Autodesk Inventor part; units mm, degrees
ref_plane "YZ Plane" through (0, 0, 0) normal (1, 0, 0) x (0, 1, 0)
ref_plane "XZ Plane" through (0, 0, 0) normal (0, 1, 0) x (-1, 0, 0)
ref_plane "XY Plane" through (0, 0, 0) normal (0, 0, 1) x (1, 0, 0)
sketch "スケッチ1" plane through (0, 0, 0) normal (0, 0, 1) x (1, 0, 0)
  line L0 (14, 16) -> (-14, 16)
  line L1 (-16, 14) -> (-16, -14)
  line L2 (-14, -16) -> (14, -16)
  line L3 (16, -14) -> (16, 14)
  line L4 (16, 16) -> (-16, -16) construction
  line L5 (-16, 16) -> (16, -16) construction
  line L6 (-13, 13) -> (13, 13) construction
  line L7 (13, 13) -> (13, -13) construction
  line L8 (13, -13) -> (-13, -13) construction
  line L9 (-13, -13) -> (-13, 13) construction
  line L10 (-13, 13) -> (13, -13) construction
  line L11 (13, 13) -> (-13, -13) construction
  circle A0 centre (-13, -13) radius 1.1
  line L12 (-16, 0) -> (16, 0) construction
  line L13 (0, 16) -> (0, -16) construction
  circle A1 centre (-13, 13) radius 1.1
  circle A2 centre (13, -13) radius 1.1
  circle A3 centre (13, 13) radius 1.1
  circle A4 centre (-13, -13) radius 2 construction
  circle A5 centre (-13, 13) radius 2 construction
  circle A6 centre (13, -13) radius 2 construction
  circle A7 centre (13, 13) radius 2 construction
  circle A8 centre (0, 0) radius 7.5
  circle A9 centre (-5.5, -9) radius 1.1
  circle A10 centre (-5.5, -9) radius 2
  line L14 (-7.5, -9) -> (-7.5, 7.5)
  line L15 (-7.5, 7.5) -> (3.5, 7.5)
  line L16 (-3.5, -9) -> (-3.5, -7.5)
  circle A11 centre (5.5, 9) radius 2
  line L17 (3.5, 9) -> (3.5, 7.5)
  circle A12 centre (5.5, 9) radius 1.1
  line L18 (7.5, 9) -> (7.5, -7.5)
  line L19 (7.5, -7.5) -> (-3.5, -7.5)
  arc A13 (-16, -14) -> (-14, -16) centre (-14, -14) ccw
  arc A14 (14, -16) -> (16, -14) centre (14, -14) ccw
  arc A15 (16, 14) -> (14, 16) centre (14, 14) ccw
  arc A16 (-14, 16) -> (-16, 14) centre (-14, 14) ccw
  line L20 (16, -11.1) -> (15, -11.1)
  line L21 (15, -11.1) -> (15, 11.1)
  line L22 (16, 11.1) -> (15, 11.1)
  point P0 (-3.5, -7.5)
  point P1 (0, -7.5)
  point P2 (-7.5, 0)
  point P3 (7.5, 0)
  point P4 (0, 7.5)
  point P5 (3.5, 7.5)
  dimension "d0" = 32
  dimension "d1" = 32
  dimension "d5" = 2.2
  dimension "d6" = 4
  dimension "d11" = 2.2
  dimension "d12" = 4
  dimension "d20" = 360
  dimension "d22" = 11
  dimension "d34" = 2
  dimension "d35" = 3
  dimension "d36" = 3
  dimension "d37" = 22.2
  dimension "d38" = 1
  dimension "d39" = 18
extrude "押し出し1" add sketch "スケッチ1" along normal blind 1.6 contours A15 L3 L22 L21 L20 A14 L2 A13 L1 A16 L0 | L3 L20 L21 L22 | A8 | L18 L19 A8 | A8 L15 L17 A11 L18 | A8 L14 L15 | L19 L16 A10 L14 A8 | A11 | A10
extrude "押し出し2" add sketch "スケッチ1" along normal blind 4.6 contours L3 L20 L21 L22
extrude "押し出し3" add sketch "スケッチ1" along normal blind 6.1 contours L18 L19 A8 | A8 L15 L17 A11 L18 | A8 L14 L15 | L19 L16 A10 L14 A8 | A11 | A10
extrude "押し出し4" add sketch "スケッチ1" along normal blind 18 contours A8
extrude "押し出し5" add sketch "スケッチ1" against normal blind 2 contours A11 | A10 | A9 | A12
properties part number "KBCR-S08MMWK"
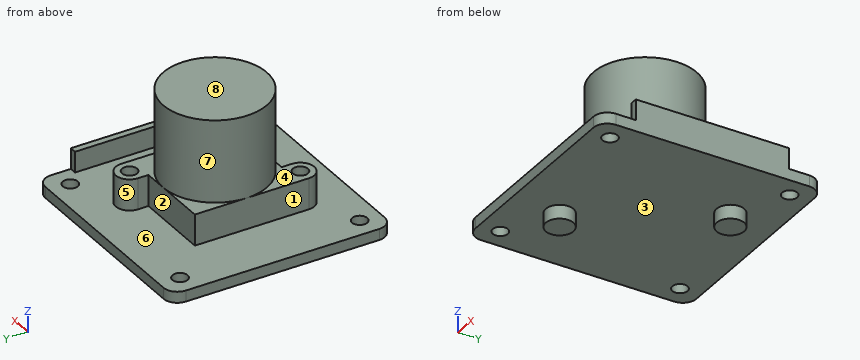
CAD build for the part. Positions are in the model's coordinates, mm. Face numbers are marked on the shaded views. A direction names the side the tool comes from. Give positions to 0.01 mm unless a question says otherwise; leave off trailing zeros. Order: outer loops, then holes, each group sorted by start corner. A loop starts at its lowest first (then second) coordinate and runs counter-clockwise, first axis right, second up. Notation, with made-up numbers: (33.25, -15) -> (38.25, -15) arc R16 cw to (38.25, 12) -> close; hole circle Ø8 at (88.5, 55). An arc over 180 degrees is marked (long way). Return JSON: item names as keys, results as strings.
Q1. Drill centre lines: line 1 (Y direction, x = 13, z = 1.5); line 2 (Y direction, x = -5.5, z = 2.75); line 3 (Z direction, x = 11.5, y = 9). Where is each one in solid material? Low to high.
Working result:
{"line 1": "-16 to -14.1, -11.9 to 11.9, 14.1 to 16", "line 2": "-11 to -10.1, -7.9 to 7.5", "line 3": "0 to 1.6"}
Q2. Flat gauge pins, fed straight in: pin 1 (10 mm diameter, centred on x = 2.5, y = -9, fed in from +Z); pin 2 (1 mm diameter, centred on x = 9.5, y = 11, fed in from -Z); pin 3 (1.5 mm diameter, centred on x = 5.5, z = 5.5, fed in from +Y); pin 4 (6 mm diameter, centred on x = -0.5, z = 15, fed in from -Y). Where does each tip first touch, or does it go through?
Working result:
{"pin 1": "z = 18", "pin 2": "z = 0", "pin 3": "y = 11", "pin 4": "y = -7.5"}
Q3. Which spindle directions (+Z, -Z, +X, -X, +Y, -Y) get a long thin tool onto all of the face, cutting with end or side? Do the marked faces 1, 2, 3, 4 and 5. Say none if no direction does.
Working result:
{"face 1": "+Z, -X, +Y, -Y", "face 2": "+Z, -X, +Y", "face 3": "-Z", "face 4": "+Z, -X, -Y", "face 5": "+Z, +Y"}
Q4. Saw through at D-D (z = 13.75). Write the cut outline in (x, y), then the cut area to 3 significant figures.
Working result:
{"outline": "circle Ø15 at (0, 0)", "area": "177 mm²"}
Q5. Saw through at A-A (x = -13). Write the cut outline in (y, z).
Working result:
{"outline": "(-16, 0) -> (-14.1, 0) -> (-14.1, 1.6) -> (-16, 1.6) -> close; (-11.9, 0) -> (11.9, 0) -> (11.9, 1.6) -> (-11.9, 1.6) -> close; (14.1, 0) -> (16, 0) -> (16, 1.6) -> (14.1, 1.6) -> close"}
Q6. Mould opens along X. For the marked faces 6, 7 and 8 say: pulls with the +X half, pulls with the -X half, needs draft (parallel to the pull), parting line crosses it, or undercut.
Working result:
{"face 6": "undercut", "face 7": "parting line crosses it", "face 8": "needs draft"}
Q7. Saw through at C-C (x = -7). Write the cut outline in (y, z).
Working result:
{"outline": "(-16, 0) -> (-10.32, 0) -> (-10.32, -2) -> (-7.68, -2) -> (-7.68, 0) -> (16, 0) -> (16, 1.6) -> (7.5, 1.6) -> (7.5, 6.1) -> (2.69, 6.1) -> (2.69, 18) -> (-2.69, 18) -> (-2.69, 6.1) -> (-10.32, 6.1) -> (-10.32, 1.6) -> (-16, 1.6) -> close"}
